from build123d import *

# Parameters (mm, degrees)
F0_W      = 40
F0_H      = 40
F0_W_2    = 35
F0_H_2    = 35
F1_DEPTH  = 100
F3_DEPTH  = 40.001
F4_DEPTH  = 40
F5_R      = 5
F6_DEPTH  = 40
F7_R      = 5
F9_DEPTH  = 2.5
F11_DEPTH = 2.5


# Not quite as in the source:
# - a feature names something its author has since deleted; it is built from what else it names


with BuildPart() as f1:
    # F0 (on Top) → F1 (new body)
    with BuildSketch(Plane.XY):
        Rectangle(F0_W, F0_H)
        Rectangle(F0_W_2, F0_H_2, mode=Mode.SUBTRACT)
    extrude(amount=F1_DEPTH)

    # F2 (on face) → F3 (cut, through all)
    with BuildSketch(Plane.YZ.offset(20)):
        with BuildLine():
            Line((20, 25.3402171373), (20, 75.7902171373))
            ThreePointArc((20, 75.7902171373), (-5.225, 50.5652171373), (20, 25.3402171373))
        make_face()
        with BuildLine():
            ThreePointArc((20, 25.3402171373), (-5.225, 50.5652171373), (20, 75.7902171373))
            Line((20, 75.7902171373), (20, 78.7902171373))
            ThreePointArc((20, 78.7902171373), (-8.225, 50.5652171373), (20, 22.3402171373))
            Line((20, 22.3402171373), (20, 25.3402171373))
        make_face()
    extrude(amount=-F3_DEPTH, mode=Mode.SUBTRACT)

    # F2 (on face) → F4 (join)
    with BuildSketch(Plane.YZ.offset(20)):
        with BuildLine():
            ThreePointArc((20, 25.3402171373), (-5.225, 50.5652171373), (20, 75.7902171373))
            Line((20, 75.7902171373), (20, 78.7902171373))
            ThreePointArc((20, 78.7902171373), (-8.225, 50.5652171373), (20, 22.3402171373))
            Line((20, 22.3402171373), (20, 25.3402171373))
        make_face()
    extrude(amount=-F4_DEPTH)

    # F5
    f5_edges = [f1.edges().sort_by_distance(p)[0] for p in [
        (-20, -20, 50),
        (20, -20, 50),
    ]]
    fillet(f5_edges, radius=F5_R)

    # F2 (on face) → F6 (cut)
    with BuildSketch(Plane.YZ.offset(20)):
        with BuildLine():
            ThreePointArc((-15, 65.9324102773), (-0.9014313771, 82.569604202), (20, 88.7902171373))
            Line((20, 88.7902171373), (20, 100))
            Line((20, 100), (-20, 100))
            Line((-20, 100), (-20, 70.5652171373))
            Line((-20, 70.5652171373), (-20, 30.5652171373))
            Line((-20, 30.5652171373), (-20, 0))
            Line((-20, 0), (20, 0))
            Line((20, 0), (20, 12.3402171373))
            ThreePointArc((20, 12.3402171373), (-0.9014313771, 18.5608300726), (-15, 35.1980239974))
            Line((-15, 35.1980239974), (-15, 65.9324102773))
        make_face()
    extrude(amount=-F6_DEPTH, mode=Mode.SUBTRACT)

    # F7
    f7_edges = [f1.edges().sort_by_distance(p)[0] for p in [
        (-20, 20, 82.290217),
        (20, 20, 82.290217),
        (-20, 20, 18.840217),
        (20, 20, 18.840217),
    ]]
    fillet(f7_edges, radius=F7_R)

    # F8 (on face) → F9 (cut)
    with BuildSketch(Plane(origin=(0, 20, 0), x_dir=(-1, 0, 0), z_dir=(0, 1, 0))):
        with BuildLine():
            ThreePointArc((0, 86.2902171373), (-4, 82.2902171373), (0, 78.2902171373))
            Line((0, 78.2902171373), (0, 86.2902171373))
        make_face()
        with BuildLine():
            Line((0, 86.2902171373), (0, 78.2902171373))
            ThreePointArc((0, 78.2902171373), (2.8284271247, 79.4617900126), (4, 82.2902171373))
            ThreePointArc((4, 82.2902171373), (2.8284271247, 85.1186442621), (0, 86.2902171373))
        make_face()
    extrude(amount=-F9_DEPTH, mode=Mode.SUBTRACT)

    # F10 (on face) → F11 (cut)
    with BuildSketch(Plane(origin=(0, 20, 0), x_dir=(-1, 0, 0), z_dir=(0, 1, 0))):
        with BuildLine():
            ThreePointArc((0, 22.8402171373), (-4, 18.8402171373), (0, 14.8402171373))
            Line((0, 14.8402171373), (0, 22.8402171373))
        make_face()
        with BuildLine():
            Line((0, 22.8402171373), (0, 14.8402171373))
            ThreePointArc((0, 14.8402171373), (2.8284271247, 16.0117900126), (4, 18.8402171373))
            ThreePointArc((4, 18.8402171373), (2.8284271247, 21.6686442621), (0, 22.8402171373))
        make_face()
    extrude(amount=-F11_DEPTH, mode=Mode.SUBTRACT)


solid = f1.part
Verification items for the finished model (mm, model axes). A direction names the side the tool comes from. Coordinates: 2 decimals unless noted, no trailing zeros. Order: outer loops, then holes, each group sorted by start corner. A loop starts at its lowest first (then second) coordinate and runs counter-clockwise, first axis right, second up.
1. Sectioned sample at A-A, the plane y = -1. Record the cut outline in (x, z).
Results found:
outline: (-20, 18.63) - (-17.5, 18.63) - (-17.5, 31.71) - (17.5, 31.71) - (17.5, 18.63) - (20, 18.63) - (20, 36.59) - (-20, 36.59) - close; (-20, 64.54) - (20, 64.54) - (20, 82.51) - (17.5, 82.51) - (17.5, 69.42) - (-17.5, 69.42) - (-17.5, 82.51) - (-20, 82.51) - close
2. Sectioned sample at B-B, the plane x = 5. Record the cut outline in (y, z) (3 decimals), and give its area (3 significant figures).
Results found:
outline: (17.5, 12.422) arc R38.225 ccw to (20, 12.34) - (20, 25.34) arc R25.225 cw to (20, 75.79) - (20, 88.79) arc R38.225 ccw to (17.5, 88.708) - (17.5, 78.679) arc R28.225 ccw to (17.5, 22.451) - close
area: 302 mm2
3. Release check for a two-part mould opening along X. For faces 4 (the face through (-20, -7, 51)), 5 (the face through (-19, -15, 50)), 6 (the face through (0, 17.5, 14)) record: +X half, -X half, draft (parallel to the pull), parting line (faces both ways), or undercut.
Results found:
face 4: -X half
face 5: draft
face 6: undercut
4. Scan lines: line 1 (X direction, y = -4.5, z = 69); line 2 (Z direction, x = 17, y = 4); line 3 (Z direction, x = 13, y = 0). Record each from-to range of solid material in increasing order.
Results found:
line 1: x = -20 to -17.5, 17.5 to 20
line 2: z = 27.31 to 31.06, 70.07 to 73.82
line 3: z = 30.65 to 35.19, 65.94 to 70.48
5. Set-up check for faces 1 (the face through (0, 17.5, 87)), 2 (the face through (17.5, -10, 50)), 3 (the face through (0, 20, 78)): record each of +Z, -Z, +X, -X, +Y, -Y from which the full face is reachable in a straight line by a thin tool's end or side.
Results found:
face 1: +Z, -Y
face 2: -Y
face 3: +Z, -Z, +X, -X, +Y
6. Sectioned sample at D-D, the plane y = 13. Record the cut outline in (x, z).
Results found:
outline: (-20, 12.99) - (-17.5, 12.99) - (-17.5, 23.22) - (17.5, 23.22) - (17.5, 12.99) - (20, 12.99) - (20, 26.33) - (-20, 26.33) - close; (-20, 74.8) - (20, 74.8) - (20, 88.14) - (17.5, 88.14) - (17.5, 77.91) - (-17.5, 77.91) - (-17.5, 88.14) - (-20, 88.14) - close
7. Sectioned sample at C-C, the plane z = 36.5. Record the cut outline in (x, y).
Results found:
outline: (-20, -15) - (-17.5, -15) - (-17.5, -4.47) - (17.5, -4.47) - (17.5, -15) - (20, -15) - (20, -0.94) - (-20, -0.94) - close
8. Go/stop test with flat-tipped pins: pin 1 Ø1 at (x, z) = (-14, 72) entering from -Y; pin 2 Ø5 at (x, z) = (-6, 15) entering from -Y; pin 3 Ø8 at (x, y) = (-14.5, -6.5) entering from +Z. Record where each tip stops, or that it passes through.
Results found:
pin 1: stops at y = 1.07
pin 2: stops at y = 17.5
pin 3: stops at z = 80.43
